Autodesk Inventor part; units mm, degrees
ref_plane "Work Plane1" through (0, 12.7, 0) normal (0, -1, 0) x (1, 0, 0)
ref_plane "YZ Plane" through (0, 0, 0) normal (1, 0, 0) x (0, 1, 0)
ref_plane "XZ Plane" through (0, 0, 0) normal (0, 1, 0) x (-1, 0, 0)
sketch "Sketch1" plane through (0, 0, 0) normal (0, 0, 1) x (1, 0, 0)
  line L0 (0, 0) -> (38.1, 0)
  line L1 (38.1, 0) -> (38.1, 25.4)
  line L2 (38.1, 25.4) -> (0, 25.4)
  line L3 (0, 25.4) -> (0, 0)
  line L4 (0, 12.7) -> (12.7, 12.7) construction
  line L5 (12.7, 12.7) -> (25.4, 12.7) construction
  circle A0 centre (12.7, 12.7) radius 2.5797
  circle A1 centre (25.4, 12.7) radius 2.5797
  dimension "d0" = 38.1
  dimension "d1" = 25.4
  dimension "d2" = 12.7
  dimension "d3" = 12.7
  dimension "d4" = 5.1594
  dimension "d5" = 5.1594
extrude "Extrusion1" add sketch "Sketch1" along normal blind 3.175
sketch "Sketch2" plane through (0, 25.4, 0) normal (0, 1, 0) x (1, 0, 0)
  circle A0 centre (41.8269, -2.2431) radius 3.175
  arc A1 (38.1, -3.0347) -> (38.7472, 0) centre (41.8269, -2.2431) ccw
  line L0 (0, 0) -> (38.1, 0)
  line L1 (38.7472, 0) -> (38.1, 0)
  line L2 (38.1, 0) -> (38.1, -3.175)
  line L3 (38.1, 0) -> (38.1, -3.175)
  dimension "d8" = 6.35
  dimension "d9" = 7.62
extrude "Extrusion2" add sketch "Sketch2" against normal blind 6.35
ref_plane "Work Plane1" through (0, 12.7, 0) normal (0, -1, 0) x (1, 0, 0)
sketch "Sketch3" plane through (0, 12.7, 0) normal (0, -1, 0) x (1, 0, 0)
  arc A0 (38.7472, 0) -> (38.1, 3.0347) centre (41.8269, 2.2431) ccw
  circle A1 centre (41.8269, 2.2431) radius 3.175
  line L0 (38.1, 0) -> (38.7472, 0)
  line L1 (38.1, 0) -> (38.1, 3.0347)
  line L2 (38.1, 3.0347) -> (38.1, 0)
  point P0 (0, 0)
extrude "Extrusion3" add sketch "Sketch3" along normal blind 6.35
properties part number "hinge"
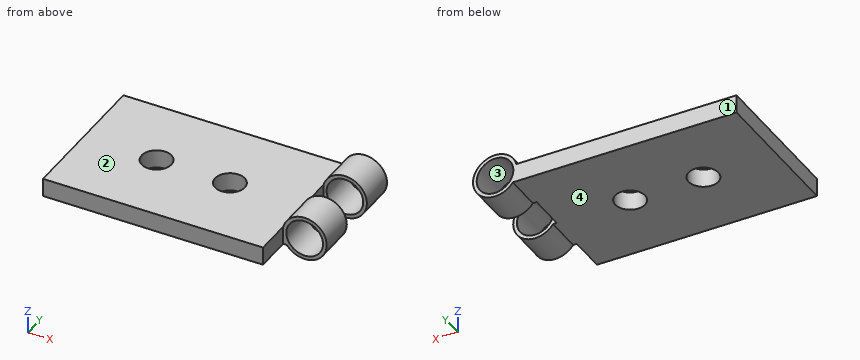
Here's how the part is built. I have some questions about the finished solid (model axes, mm). Face numbers are marked on the shaded views. A direction names the side the tool comes from. Round coordinates to 2 decimals unless told otherwise and drop trailing zeros. Order: outer loops, then holes, each group sorted by start corner. A loop starts at its lowest first (then second) coordinate and runs counter-clockwise, first axis right, second up. Notation, with made-up numbers: (41.25, -2.5) -> (61.25, -2.5) arc R8 ccw to (61.25, 9.5) -> close; hole circle Ø5 at (-4, 34.5). An arc over 180 degrees is marked (long way). Return JSON: item names as keys, results as strings.
Q1. Which directions (+Z, -Z, +X, -X, +Y, -Y) give clear straight access to the entire face, cutting with the end or side of a thin tool? Please do the marked faces 1 and 2.
Filled sheet:
{"face 1": "+Z, -Z, +X, -X, +Y", "face 2": "+Z, -X, +Y, -Y"}
Q2. If we section it at A-A on x = 12.7: List the corners of the cut face in (y, z) for me (3 decimals).
Filled sheet:
{"outline": "(0, 0) -> (10.12, 0) -> (10.12, 3.175) -> (0, 3.175) -> close; (15.28, 0) -> (25.4, 0) -> (25.4, 3.175) -> (15.28, 3.175) -> close"}
Q3. If we mould it in two halves opening along X, with no side actions, what happens to the marked faces 3 and 4? For each: released by +X, released by -X, zero draft, split by the parting line, or undercut.
Filled sheet:
{"face 3": "undercut", "face 4": "zero draft"}
Q4. I need wall thicknesses on line 1 along X through (y, z) = (24.5, 2); line 2 along Y through (x, z) = (25.4, 1.75); line 3 along X through (y, z) = (14.5, 2.5). Which ranges of each line are inside material? Lowest first, please. Write a range as from..to.
Filled sheet:
{"line 1": "x = 0..38.66, 44.99..45.63", "line 2": "y = 0..10.12, 15.28..25.4", "line 3": "x = 0..10.85, 14.55..23.55, 27.25..38.1"}
Q5. If we section it at B-B on y = 11.75: List the corners of the cut face in (x, z) for me (3 decimals).
Filled sheet:
{"outline": "(0, 0) -> (10.302, 0) -> (10.302, 3.175) -> (0, 3.175) -> close; (15.098, 0) -> (23.002, 0) -> (23.002, 3.175) -> (15.098, 3.175) -> close; (27.798, 0) -> (38.747, 0) arc R3.81 ccw (long way) to (38.1, 3.035) -> (38.1, 3.175) -> (27.798, 3.175) -> close; hole circle Ø6.35 at (41.827, 2.243)"}
Q6. For pin 1 Ø6.5 at (x, y) = (25.4, 12.7) entering from -Z; pin 2 Ø2.5 at (y, z) = (8.5, 1.5) entering from +X; pin 3 Ø12.5 at (x, y) = (20, 13.5) entering from +Z (3 decimals); pin 4 Ø1.5 at (x, y) = (39, 22.5) entering from +Z, each with a flat end and sliding along its axis, tell me the tip position at first contact or that it passes through.
Filled sheet:
{"pin 1": "stops at z = 0", "pin 2": "stops at x = 45.64", "pin 3": "stops at z = 3.175", "pin 4": "stops at z = 5.44"}
Q7. If we section it at C-C on z = 4.25: List the corners of the cut face in (x, y) for me.
Filled sheet:
{"outline": "(38.59, 6.35) -> (39.37, 6.35) -> (39.37, 12.7) -> (38.59, 12.7) -> close; (38.59, 19.05) -> (39.37, 19.05) -> (39.37, 25.4) -> (38.59, 25.4) -> close; (44.29, 6.35) -> (45.07, 6.35) -> (45.07, 12.7) -> (44.29, 12.7) -> close; (44.29, 19.05) -> (45.07, 19.05) -> (45.07, 25.4) -> (44.29, 25.4) -> close"}
Q8. If we section it at D-D on y = 23.75: List the corners of the cut face in (x, z) for me (3 decimals), plus the area to 3 significant figures.
Filled sheet:
{"outline": "(0, 0) -> (38.747, 0) arc R3.81 ccw (long way) to (38.1, 3.035) -> (38.1, 3.175) -> (0, 3.175) -> close; hole circle Ø6.35 at (41.827, 2.243)", "area": "135 mm^2"}
